from build123d import *

# Parameters (mm, degrees)
SKETCH1_R           = 9.652
BOSS_EXTRUDE1_DEPTH = 3.302
SKETCH1_4_R         = 4.826
BOSS_EXTRUDE2_DEPTH = 130.302
SKETCH1_6_R         = 3.302
CUT_EXTRUDE1_DEPTH  = 127


with BuildPart() as part:
    # Sketch1 → Boss-Extrude1 (new body)
    with BuildSketch(Plane(origin=(0, 0, 0), x_dir=(1, 0, 0), z_dir=(0, 1, 0))):
        with Locations(Location((0, 0, 0), (0, 0, 90))):
            Circle(SKETCH1_R)
    extrude(amount=BOSS_EXTRUDE1_DEPTH)

    # Sketch1_4 → Boss-Extrude2 (add)
    with BuildSketch(Plane(origin=(0, 0, 0), x_dir=(1, 0, 0), z_dir=(0, 1, 0))):
        with Locations(Location((0, 0, 0), (0, 0, 270))):
            Circle(SKETCH1_4_R)
    extrude(amount=BOSS_EXTRUDE2_DEPTH)

    # Sketch1_6 → Cut-Extrude1 (cut)
    with BuildSketch(Plane(origin=(0, 0, 0), x_dir=(1, 0, 0), z_dir=(0, 1, 0))):
        with Locations(Location((0, 0, 0), (0, 0, 270))):
            Circle(SKETCH1_6_R)
    extrude(amount=CUT_EXTRUDE1_DEPTH, mode=Mode.SUBTRACT)


solid = part.part
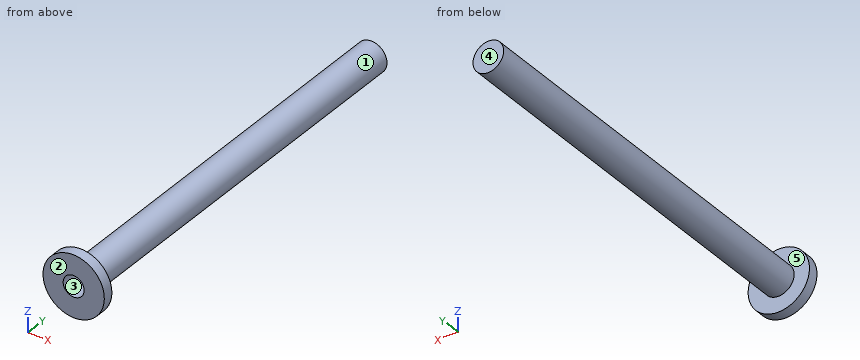
The model under review builds one solid part; all positions refer to its coordinate system, in mm. Face numbers are marked on the shaded views. A direction names the side the tool comes from. Coordinates: 2 decimals unless noted, no trailing zeros. Loops run counter-clockwise (first coordinate to the right, second up) from the corner with the lowest first, then second, coordinate; pieces in that order, holes last.
(1) Draft analysis for pull direction Z (two halves, no side actions). For the marked faces 1, 2 and 3, state which applies: +Z half, -Z half, draft (parallel to the pull), parting line (faces both ways), or undercut.
Determined:
face 1: parting line
face 2: draft
face 3: undercut
(2) Consider section B-B, the plane z = 0. Give the boundary of the cut face in (x, y), plus the area to 3 significant figures.
Determined:
outline: (-9.65, 0) - (-3.3, 0) - (-3.3, 127) - (3.3, 127) - (3.3, 0) - (9.65, 0) - (9.65, 3.3) - (4.83, 3.3) - (4.83, 130.3) - (-4.83, 130.3) - (-4.83, 3.3) - (-9.65, 3.3) - close
area: 451 mm2
(3) Consider section C-C, the plane y = 22. Give the boundary of the cut face in (x, z).
Determined:
outline: circle Ø9.65 at (0, 0); hole circle Ø6.6 at (0, 0)
(4) Wall thickness on L1, parallel to X at y = 109, z = 0; L2, parallel to Z at x = 0.75, y = 56.5; L3, parallel to Y at x = 1.75, z = -7.5: over which ranges is each line inside the solid? List them lowest first.
Determined:
L1: x = -4.83 to -3.3, 3.3 to 4.83
L2: z = -4.77 to -3.22, 3.22 to 4.77
L3: y = 0 to 3.3
(5) Insertion check: P1, Ø8, axis at y = 74, z = 0, coming from the +X side; P2, Ø2, axis at x = -6, y = 92.5, coming from the -Z side (1 decimal); P3, Ø5.5, axis at x = -0.5, z = 0, coming from the -Y side; P4, Ø1, axis at x = 6.5, z = 7, coming from the +Y side. Each pin has a flat end and moves straight along its axis. Give the tip position at first contact, or say it passes through.
Determined:
P1: stops at x = 4.83
P2: passes through
P3: stops at y = 127
P4: stops at y = 3.3
(6) Tool access review of the marked faces 4 and 5: name each direction out of +Z, -Z, +X, -X, +Y, -Y from which nothing blocks a thin tool from reaching the whole face with its end or side.
Determined:
face 4: +Z, -Z, +X, -X, +Y
face 5: +Y
(7) Consider section A-A, the plane x = 0. Give the boundary of the cut face in (y, z), plus the area to 3 significant figures.
Determined:
outline: (0, -9.65) - (3.3, -9.65) - (3.3, -4.83) - (130.3, -4.83) - (130.3, 4.83) - (3.3, 4.83) - (3.3, 9.65) - (0, 9.65) - (0, 3.3) - (127, 3.3) - (127, -3.3) - (0, -3.3) - close
area: 451 mm2
(8) Consider section D-D, the plane x = -8.5. Give the boundary of the cut face in (y, z), plus the area to 3 significant figures.
Determined:
outline: (0, -4.57) - (3.3, -4.57) - (3.3, 4.57) - (0, 4.57) - close
area: 30.2 mm2
